Autodesk Inventor part; units mm, degrees
ref_plane "YZ Plane" through (0, 0, 0) normal (1, 0, 0) x (0, 1, 0)
ref_plane "XZ Plane" through (0, 0, 0) normal (0, 1, 0) x (-1, 0, 0)
ref_plane "XY Plane" through (0, 0, 0) normal (0, 0, 1) x (1, 0, 0)
sketch "Sketch1" plane through (0, 0, 0) normal (0, 1, 0) x (-1, 0, 0)
  circle A0 centre (0, 0) radius 25
  line L0 (25, 0) -> (25, -208.3553)
  line L1 (25, -208.3553) -> (-34.3223, -267.6777)
  line L2 (-25, 0) -> (-25, -187.6447)
  line L3 (-25, -187.6447) -> (-69.6777, -232.3223)
  circle A1 centre (-52, -250) radius 25
  dimension "d0" = 50
  dimension "d1" = 50
  dimension "d2" = 250
  dimension "d3" = 27
  dimension "d4" = 135
extrude "Extrusion1" add sketch "Sketch1" along normal blind 30
sketch "Sketch2" plane through (0, 0, 0) normal (0, -1, 0) x (1, 0, 0)
  line L0 (-10, -36) -> (10, -36)
  line L1 (10, -36) -> (10, 18)
  line L2 (10, 18) -> (-10, 18)
  line L3 (-10, 18) -> (-10, -36)
  line L4 (-10, -29) -> (10, -29)
  line L5 (10, -29) -> (10, 11)
  line L6 (10, 11) -> (-10, 11)
  line L7 (-10, 11) -> (-10, -29)
  point P0 (0, 0)
  point P1 (-10, 11)
  dimension "d7" = 54
  dimension "d8" = 20
  dimension "d9" = 10
  dimension "d10" = 7
  dimension "d11" = 40
  dimension "d12" = 36
extrude "Extrusion2" cut sketch "Sketch2" against normal through all contours L3 L6 L1 L4
sketch "Sketch3" plane through (0, 30, 0) normal (0, 1, 0) x (1, 0, 0)
  line L0 (-10, -18) -> (10, -18)
  line L1 (10, -18) -> (10, 36)
  line L2 (10, 36) -> (-10, 36)
  line L3 (-10, 36) -> (-10, -18)
  line L4 (10, -11) -> (-10, -11)
  line L5 (-10, 29) -> (10, 29)
  point P0 (0, 0)
  dimension "d15" = 7
  dimension "d16" = 7
extrude "Extrusion3" cut sketch "Sketch3" against normal blind 21 contours L3 L4 L1 L0 | L3 L2 L1 L5
sketch "Sketch4" plane through (0, 30, 0) normal (0, 1, 0) x (1, 0, 0)
  point P0 (0, 0)
properties part number "Arm 1"
Geometry: final body of the model. Coordinates: model frame, mm. A direction names the side the tool comes from. Give positions to 0.01 mm unless a question says otherwise; leave off trailing zeros. Loops run counter-clockwise (first coordinate to the right, second up) from the corner with the lowest first, then second, coordinate; pieces in that order, holes last. Notation, with made-up numbers: (-18.75, 5) -> (21.25, 5) arc R27 cw to (21.25, 38) -> close; hole circle Ø4 at (72.5, 24). An arc over 180 degrees is marked (long way). Put each result on its own line as item: value.
1. Ray query, line 1 along X through (y, z) = (16.5, -3); line 2 along X through (y, z) = (11, -119); line 3 along X through (y, z) = (7, -197). Return the intervals inside material, ascending. Write a range as [from, to].
Taken from the geometry:
line 1: x = [-25, -10], [10, 25]
line 2: x = [-25, 25]
line 3: x = [-25, 34.36]
2. Cut plane C-C (z = -78). Return the cut outline in (x, y).
Taken from the geometry:
outline: (-25, 0) -> (25, 0) -> (25, 30) -> (-25, 30) -> close
3. Pull-direction query (X, two-part tool) for faces 6 (the cylindrical face through (69.285, 14.79, -268.062)), 7 (the flat face through (10, 15, -9)), 8 (the flat face through (4.246, 14.79, -237.601)); classes: released by +X, released by -X, zero draft, split by the parting line, or undercut.
Taken from the geometry:
face 6: split by the parting line
face 7: undercut
face 8: released by -X
4. Cut plane D-D (y = 17.75). Return the cut outline in (x, z), plus the area to 3 significant figures.
Taken from the geometry:
outline: (-25, -208.36) -> (34.32, -267.68) arc R25 ccw to (69.68, -232.32) -> (25, -187.64) -> (25, 0) arc R25 ccw to (-25, 0) -> close; hole (-10, -36) -> (10, -36) -> (10, 18) -> (-10, 18) -> close
area: 14,500 mm2
5. Cut plane A-A (x = 6.5). Return the cut outline in (y, z), plus the area to 3 significant figures.
Taken from the geometry:
outline: (0, -239.86) -> (30, -239.86) -> (30, -36) -> (9, -36) -> (9, -29) -> (0, -29) -> close; (0, 11) -> (9, 11) -> (9, 18) -> (30, 18) -> (30, 24.14) -> (0, 24.14) -> close
area: 6,430 mm2
6. Pin query (flat end, axial travel): P1, Ø15, axis at y = 17.5, z = -21, coming from the +X side; P2, Ø10, axis at x = 4, y = 5, coming from the -Z side; P3, Ø5.5, axis at x = -1.5, z = -33, coming from the +Y side. Return the tip coordinate at first contact, or that it passes through.
Taken from the geometry:
P1: stops at x = 25
P2: stops at z = -242.36
P3: stops at y = 9
7. Cut plane B-B (y = 5.75). Return the cut outline in (x, z), plus the area to 3 significant figures.
Taken from the geometry:
outline: (-25, -208.36) -> (34.32, -267.68) arc R25 ccw to (69.68, -232.32) -> (25, -187.64) -> (25, 0) arc R25 ccw to (-25, 0) -> close; hole (-10, -29) -> (10, -29) -> (10, 11) -> (-10, 11) -> close
area: 14,700 mm2
8. Set-up query: faces 1 (the flat face through (25, 15, -93)), 2 (the flat face through (15, 30, -156)), 3 (the flat face through (0, 4, -29)), 4 (the flat face through (-25, 15, -103)), 5 (the flat face through (0, 20, -36)). Return all of +Z, -Z, +X, -X, +Y, -Y with unobstructed straight access to the full face (end or side cutting, diameter ignored); none if empty.
Taken from the geometry:
face 1: +Z, +X, +Y, -Y
face 2: +Z, -Z, +X, -X, +Y
face 3: +Y, -Y
face 4: +Z, -Z, -X, +Y, -Y
face 5: +Y
